The listing builds one solid part. Answer for the finished solid, in the listing's coordinates (mm). A direction names the side the tool comes from. Round coordinates to 2 decimals unless told otherwise and drop trailing zeros. Loops run counter-clockwise (first coordinate to the right, second up) from the corner with the lowest first, then second, coordinate; pieces in that order, holes last. Notation, with made-up numbers: M -5,15.25 L 9,15.25 A16 cw 9,43.25 Z; hole C 77,7 d3. An arc over 180 degrees is marked long. Answer as a JSON object with one key per item and string values.
```python
from build123d import *

# Parameters (mm, degrees)
SKETCH1_R           = 4
SKETCH1_W           = 0.443674292
SKETCH1_H           = 0.606573965
SKETCH1_W_2         = 0.441272097
SKETCH1_W_3         = 0.539332563
SKETCH1_W_4         = 0.547504268
SKETCH1_W_5         = 0.686423262
SKETCH1_W_6         = 0.607984695
SKETCH1_W_7         = 0.472854348
SKETCH1_W_8         = 0.501804613
SKETCH1_W_9         = 0.559705146
SKETCH1_W_10        = 0.321886919
SKETCH1_W_11        = 0.335329484
BOSS_EXTRUDE1_DEPTH = 36.8
SKETCH2_W           = 17.119195375
SKETCH2_H           = 26.8
CUT_EXTRUDE1_DEPTH  = 45


with BuildPart() as part:
    # Sketch1 → Boss-Extrude1 (new body)
    with BuildSketch(Plane.XY):
        with BuildLine():
            ThreePointArc((-2.487228681, 2.47588145), (-1.643417841, 0.836304882), (0, 0))
            Line((0, 0), (42.98, -6.863043607))
            ThreePointArc((42.98, -6.863043607), (44.726436776, -6.986706153), (46.46767433, -6.803879411))
            ThreePointArc((46.46767433, -6.803879411), (60.333502735, -6.411334854), (73.586869705, -10.505666612))
            ThreePointArc((73.586869705, -10.505666612), (75.109024375, -11.116277731), (76.710514264, -11.469874834))
            Line((76.710514264, -11.469874834), (76.710514264, -10.954571675))
            Line((76.710514264, -10.954571675), (77.19406036, -10.954571675))
            Line((77.19406036, -10.954571675), (77.47538128, -10.954571675))
            Line((77.47538128, -10.954571675), (77.981998439, -10.954571675))
            Line((77.981998439, -10.954571675), (78.200260874, -10.954571675))
            Line((78.200260874, -10.954571675), (78.643935166, -10.954571675))
            Line((78.643935166, -10.954571675), (78.872742919, -10.954571675))
            Line((78.872742919, -10.954571675), (79.314015016, -10.954571675))
            Line((79.314015016, -10.954571675), (79.591853003, -10.954571675))
            Line((79.591853003, -10.954571675), (80.131185566, -10.954571675))
            Line((80.131185566, -10.954571675), (80.343649909, -10.954571675))
            Line((80.343649909, -10.954571675), (80.891154177, -10.954571675))
            Line((80.891154177, -10.954571675), (81.013729759, -10.954571675))
            Line((81.013729759, -10.954571675), (81.700153021, -10.954571675))
            Line((81.700153021, -10.954571675), (81.871758836, -10.954571675))
            Line((81.871758836, -10.954571675), (82.419263104, -10.954571675))
            Line((82.419263104, -10.954571675), (82.535057995, -10.954571675))
            Line((82.535057995, -10.954571675), (83.14304269, -10.954571675))
            Line((83.14304269, -10.954571675), (83.326547781, -10.954571675))
            Line((83.326547781, -10.954571675), (83.799402129, -10.954571675))
            Line((83.799402129, -10.954571675), (84.002053992, -10.954571675))
            Line((84.002053992, -10.954571675), (84.503858605, -10.954571675))
            Line((84.503858605, -10.954571675), (84.677560202, -10.954571675))
            Line((84.677560202, -10.954571675), (85.237265348, -10.954571675))
            Line((85.237265348, -10.954571675), (85.365140123, -10.954571675))
            Line((85.365140123, -10.954571675), (85.700469607, -10.954571675))
            Line((85.700469607, -10.954571675), (85.806620583, -10.954571675))
            Line((85.806620583, -10.954571675), (86.128507502, -10.954571675))
            Line((86.128507502, -10.954571675), (86.128507502, -11.56114564))
            ThreePointArc((86.128507502, -11.56114564), (88.510189101, -10.385314701), (89.024900759, -7.779540815))
            Line((89.024900759, -7.779540815), (88.261533379, -4.950730067))
            ThreePointArc((88.261533379, -4.950730067), (88.089699744, -4.476637927), (87.840885143, -4.038024828))
            Line((87.840885143, -4.038024828), (78.200260874, 10.048964336))
            ThreePointArc((78.200260874, 10.048964336), (73.431103782, 15.477008911), (67.502436306, 19.607315102))
            Line((67.502436306, 19.607315102), (21.566587187, 43.977332864))
            ThreePointArc((21.566587187, 43.977332864), (14.751147415, 46.588108627), (7.506961555, 47.47588145))
            Line((7.506961555, 47.47588145), (1.426961555, 47.47588145))
            ThreePointArc((1.426961555, 47.47588145), (0.761339604, 47.401107495), (0.128898443, 47.180513062))
            ThreePointArc((0.128898443, 47.180513062), (-1.383603673, 46.332621816), (-2.77660534, 45.300086793))
            ThreePointArc((-2.77660534, 45.300086793), (-6.782062218, 39.585860112), (-7.445250004, 32.639188007))
            Line((-7.445250004, 32.639188007), (-2.487228681, 2.47588145))
        make_face()
        with Locations((8.267526818, 9.561727541)):
            Circle(SKETCH1_R, mode=Mode.SUBTRACT)
        with Locations((3.948380067, 39.69588145)):
            Circle(SKETCH1_R, mode=Mode.SUBTRACT)
        with BuildLine():
            Line((76.710514264, -10.954571675), (76.710514264, -11.469874834))
            ThreePointArc((76.710514264, -11.469874834), (76.951959843, -11.499734689), (77.19406036, -11.523712134))
            Line((77.19406036, -11.523712134), (77.19406036, -10.954571675))
            Line((77.19406036, -10.954571675), (76.710514264, -10.954571675))
        make_face()
        with BuildLine():
            Line((77.47538128, -10.954571675), (77.47538128, -11.544129353))
            ThreePointArc((77.47538128, -11.544129353), (77.728583879, -11.555701678), (77.981998439, -11.560852954))
            Line((77.981998439, -11.560852954), (77.981998439, -10.954571675))
            Line((77.981998439, -10.954571675), (77.47538128, -10.954571675))
        make_face()
        with Locations((78.42209802, -11.257858658)):
            Rectangle(SKETCH1_W, SKETCH1_H)
        with Locations((79.093378968, -11.257858658)):
            Rectangle(SKETCH1_W_2, SKETCH1_H)
        with Locations((79.861519285, -11.257858658)):
            Rectangle(SKETCH1_W_3, SKETCH1_H)
        with Locations((80.617402043, -11.257858658)):
            Rectangle(SKETCH1_W_4, SKETCH1_H)
        with Locations((81.35694139, -11.257858658)):
            Rectangle(SKETCH1_W_5, SKETCH1_H)
        with Locations((82.14551097, -11.257858658)):
            Rectangle(SKETCH1_W_4, SKETCH1_H)
        with Locations((82.839050343, -11.257858658)):
            Rectangle(SKETCH1_W_6, SKETCH1_H)
        with Locations((83.562974955, -11.257858658)):
            Rectangle(SKETCH1_W_7, SKETCH1_H)
        with Locations((84.252956299, -11.257858658)):
            Rectangle(SKETCH1_W_8, SKETCH1_H)
        with Locations((84.957412775, -11.257858658)):
            Rectangle(SKETCH1_W_9, SKETCH1_H)
        with Locations((85.967564043, -11.257858658)):
            Rectangle(SKETCH1_W_10, SKETCH1_H)
        with Locations((85.532804865, -11.257858658)):
            Rectangle(SKETCH1_W_11, SKETCH1_H)
    extrude(amount=BOSS_EXTRUDE1_DEPTH)

    # Sketch2 → Cut-Extrude1 (cut)
    with BuildSketch(Plane(origin=(0, -40, 0), x_dir=(1, 0, 0), z_dir=(0, 1, 0))):
        with Locations((60.027272017, -18.4)):
            Rectangle(SKETCH2_W, SKETCH2_H)
    extrude(amount=CUT_EXTRUDE1_DEPTH, mode=Mode.SUBTRACT)


solid = part.part
```
Item 1: The part is cut by section A-A (y = 41.5). Give the vertices of the cut face in (x, z), then the cut area to 3 significant figures.
Values follow:
{"outline": "M -5.9,0 L 0.38,0 L 0.38,36.8 L -5.9,36.8 Z; M 7.52,0 L 26.24,0 L 26.24,36.8 L 7.52,36.8 Z", "area": "920 mm^2"}
Item 2: The part is cut by section B-B (y = -3). Give the vertices of the cut face in (x, z), then the cut area to 3 significant figures.
Values follow:
{"outline": "M 18.79,0 L 87.13,0 L 87.13,36.8 L 18.79,36.8 Z; hole M 51.47,5 L 68.59,5 L 68.59,31.8 L 51.47,31.8 Z", "area": "2,060 mm^2"}
Item 3: The part is cut by section D-D (y = 8). Give the vertices of the cut face in (x, z) (1 decimal), then the cut area to 3 significant figures.
Values follow:
{"outline": "M -3.4,0 L 4.6,0 L 4.6,36.8 L -3.4,36.8 Z; M 12,0 L 79.6,0 L 79.6,36.8 L 12,36.8 Z", "area": "2,780 mm^2"}
Item 4: The part is cut by section C-C (z = 33). Give the number of separate pieces and of enclosed holes in the cut face, then the cut area to 3 significant figures.
Values follow:
{"separate pieces": "1", "enclosed holes": "2", "area": "3,330 mm^2"}
Item 5: Which of the six approach directions +Z, -Z, +X, -X, +Y, -Y give full straight-line access (tool end or side, diameter ignored) to faces 1 (the face through (5, 47.476, 18)), 2 (the face through (68.587, -2, 19))?
Values follow:
{"face 1": "+Z, -Z, +X, -X, +Y", "face 2": "-Y"}
Item 6: Straight lines are drawn through the part: line 1 (Y direction, x = 5, z = 26.5); line 2 (X direction, y = 41, z = 34.5); line 3 (Y direction, x = 18.5, z = 7). For each, find the intervals that lie inside material, in ascending order.
Values follow:
{"line 1": "-0.8 to 7.25, 11.87 to 35.84, 43.56 to 47.48", "line 2": "-6.17 to 0.17, 7.73 to 27.18", "line 3": "-2.95 to 45.39"}
Item 7: Flat-ended cylindrical pins translate along their axes: P1, Ø1.5, axis at y = 0.5, z = 27, coming from the +X side; P2, Ø0.7, axis at y = -11.5, z = 24.5, coming from the +X side; P3, Ø0.7, axis at y = -11, z = 17, coming from the -X side. Find the tip coordinate at first contact, or state that the pin passes through.
Values follow:
{"P1": "x = 85.25", "P2": "x = 87.64", "P3": "x = 73.89"}
Item 8: Determine the mould class of faces 3 (the face through (73.507, 15.409, 18.142)), 4 (the face through (60, 5, 18)), 5 (the face through (29, 18, 36.8)) for opening direction Z: released by +Z, released by -Z, zero draft, split by the parting line, or undercut.
Values follow:
{"face 3": "zero draft", "face 4": "undercut", "face 5": "released by +Z"}
